from build123d import *

# Parameters (mm, degrees)
SKETCH_R      = 3.9
SKETCH_R_2    = 2.6
PAD_DEPTH     = 5
SKETCH001_R   = 8
SKETCH001_R_2 = 2.6
PAD001_DEPTH  = 3
CHAMFER_SIZE  = 1


with BuildPart() as part:
    # Sketch → Pad (new body)
    with BuildSketch(Plane.XY):
        Circle(SKETCH_R)
        Circle(SKETCH_R_2, mode=Mode.SUBTRACT)
    extrude(amount=PAD_DEPTH)

    # Sketch001 (on Face4 of Pad) → Pad001 (join)
    with BuildSketch(Plane.XY.offset(5)):
        Circle(SKETCH001_R)
        Circle(SKETCH001_R_2, mode=Mode.SUBTRACT)
    extrude(amount=PAD001_DEPTH)

    # Chamfer
    chamfer_edges = [part.edges().sort_by_distance(p)[0] for p in [
        (-8, 0, 5),
    ]]
    chamfer(chamfer_edges, length=CHAMFER_SIZE)


solid = part.part
Build history of the part. All positions in model axes, mm. A direction names the side the tool comes from. Coordinates: 2 decimals unless noted, no trailing zeros. Write each loop counter-clockwise with the first axis right and the second up, starting at its lowest first coordinate (ties: lowest second). Pieces come first, ordered by that corner, then holes.
(1) Pin check, flat tips, straight feed: pin 1 Ø1 at (x, z) = (3, 2) entering from +Y; pin 2 Ø2 at (x, z) = (5.5, 4.5) entering from +Y; pin 3 Ø3 at (x, z) = (-2, 6) entering from +Y. Stop position of each tip, or through.
(2) 3-axis set-ups, long thin cutter, end or side, ignore diameter. For faces 4 (the flat face through (3, -1, 0)), 5 (the cylindrical face through (-2.87, 2.64, 2.46)): which of +Z, -Z, +X, -X, +Y, -Y reach the whole face in a straight line?
(3) Mould opens along Y. For faces 1 (the cylindrical face through (-1.73, -7.81, 6.99)), 2 (the flat face through (3, -3, 5)), 3 (the cylindrical face through (-0.338, 2.578, 3.944)) say: pulls with the +Y half, pulls with the -Y half, needs draft (parallel to the pull), parting line crosses it, or undercut.
(4) Cut at C-C on z = 2. List the corners of the cut face in (x, y).
(5) Drill centre lines: line 1 (Y direction, x = 0, z = 4.75); line 2 (Z direction, x = -1.25, y = 6.5); line 3 (X direction, y = -2.25, z = 1.25). Where is each one in solid material? Low to high.
(6) Cut at A-A on x = 0. List the corners of the cut face in (y, z).
Working result:
1. pin 1: stops at y = 2.99
1. pin 2: stops at y = 5.41
1. pin 3: stops at y = 7.98
2. face 4: -Z, +X, -X, +Y, -Y
2. face 5: -Z
3. face 1: parting line crosses it
3. face 2: needs draft
3. face 3: undercut
4. outline: circle Ø7.8 at (0, 0); hole circle Ø5.2 at (0, 0)
5. line 1: y = -3.9 to -2.6, 2.6 to 3.9
5. line 2: z = 5 to 8
5. line 3: x = -3.19 to -1.3, 1.3 to 3.19
6. outline: (-8, 6) - (-7, 5) - (-3.9, 5) - (-3.9, 0) - (-2.6, 0) - (-2.6, 8) - (-8, 8) - close; (2.6, 0) - (3.9, 0) - (3.9, 5) - (7, 5) - (8, 6) - (8, 8) - (2.6, 8) - close
